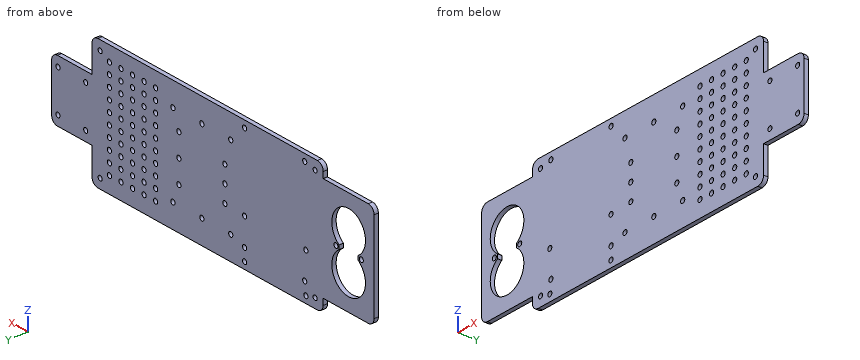
from build123d import *

# Parameters (mm, degrees)
SKETCH1_W           = 200
SKETCH1_H           = 95
BOSS_EXTRUDE1_DEPTH = 3.175
SKETCH3_R           = 1.75
CUT_EXTRUDE2_DEPTH  = 118.785400915
SKETCH4_W           = 76
SKETCH4_H           = 3.175
BOSS_EXTRUDE2_DEPTH = 44
SKETCH5_R           = 1.75
CUT_EXTRUDE3_DEPTH  = 148.223024992
SKETCH7_W           = 45
SKETCH7_H           = 3.175
BOSS_EXTRUDE3_DEPTH = 35
SKETCH8_R           = 1.75
CUT_EXTRUDE4_DEPTH  = 151.064564226
FILLET1_R           = 5
SKETCH9_R           = 1.775
CUT_EXTRUDE5_DEPTH  = 151.064564226
SKETCH10_R          = 1.8
SKETCH10_R_2        = 1.775
CUT_EXTRUDE6_DEPTH  = 151.064564226
SKETCH11_R          = 1.8
CUT_EXTRUDE7_DEPTH  = 151.064564226
SKETCH12_R          = 1.8
CUT_EXTRUDE8_DEPTH  = 151.064564226


with BuildPart() as part:
    # Sketch1 → Boss-Extrude1 (new body)
    with BuildSketch(Plane(origin=(0, 0, 0), x_dir=(1, 0, 0), z_dir=(0, 1, 0))):
        with Locations((6.013896682, 3.728641929)):
            Rectangle(SKETCH1_W, SKETCH1_H)
    extrude(amount=BOSS_EXTRUDE1_DEPTH)

    # Sketch3 → Cut-Extrude2 (cut, through all)
    with BuildSketch(Plane(origin=(0, 3.175, 0), x_dir=(1, 0, 0), z_dir=(0, 1, 0))):
        with Locations(Location((-86.986103318, -36.771358071, 0), (0, 0, 270))):
            Circle(SKETCH3_R)
        with Locations(Location((-86.986103318, 44.228641929, 0), (0, 0, 270))):
            Circle(SKETCH3_R)
        with Locations(Location((99.013896682, 44.228641929, 0), (0, 0, 270))):
            Circle(SKETCH3_R)
        with Locations(Location((99.013896682, -36.771358071, 0), (0, 0, 270))):
            Circle(SKETCH3_R)
    extrude(amount=-CUT_EXTRUDE2_DEPTH, mode=Mode.SUBTRACT)

    # Sketch4 → Boss-Extrude2 (add)
    with BuildSketch(Plane.ZY.offset(93.986103318)):
        with Locations((-3.728641929, 1.5875)):
            Rectangle(SKETCH4_W, SKETCH4_H)
    extrude(amount=BOSS_EXTRUDE2_DEPTH)

    # Sketch5 → Cut-Extrude3 (cut, through all)
    with BuildSketch(Plane(origin=(0, 3.175, 0), x_dir=(1, 0, 0), z_dir=(0, 1, 0))):
        with Locations(Location((-126.986103318, 3.728641929, 0), (0, 0, 270))):
            Circle(SKETCH5_R)
        with Locations(Location((-104.986103318, 3.728641929, 0), (0, 0, 270))):
            Circle(SKETCH5_R)
        with BuildLine():
            Line((-124.286103318, 2.179060332), (-124.286103318, 5.278223526))
            ThreePointArc((-124.286103318, 5.278223526), (-115.986103318, 31.778641929), (-107.686103318, 5.278223526))
            Line((-107.686103318, 5.278223526), (-107.686103318, 2.179060332))
            ThreePointArc((-107.686103318, 2.179060332), (-115.986103318, -24.321358071), (-124.286103318, 2.179060332))
        make_face()
    extrude(amount=-CUT_EXTRUDE3_DEPTH, mode=Mode.SUBTRACT)

    # Sketch7 → Boss-Extrude3 (add)
    with BuildSketch(Plane(origin=(106.013896682, 0, 0), x_dir=(0, 0, -1), z_dir=(1, 0, 0))):
        with Locations((3.728641929, 1.5875)):
            Rectangle(SKETCH7_W, SKETCH7_H)
    extrude(amount=BOSS_EXTRUDE3_DEPTH)

    # Sketch8 → Cut-Extrude4 (cut, through all)
    with BuildSketch(Plane(origin=(0, 3.175, 0), x_dir=(1, 0, 0), z_dir=(0, 1, 0))):
        with Locations(Location((111.513896682, -11.471358071, 0), (0, 0, 270))):
            Circle(SKETCH8_R)
        with Locations(Location((111.513896682, 18.928641929, 0), (0, 0, 270))):
            Circle(SKETCH8_R)
        with Locations(Location((135.513896682, -11.471358071, 0), (0, 0, 270))):
            Circle(SKETCH8_R)
        with Locations(Location((135.513896682, 18.928641929, 0), (0, 0, 270))):
            Circle(SKETCH8_R)
    extrude(amount=-CUT_EXTRUDE4_DEPTH, mode=Mode.SUBTRACT)

    # Fillet1
    fillet1_edges = [part.edges().sort_by_distance(p)[0] for p in [
        (106.013896682, 1.5875, -51.228641929),
        (141.013896682, 1.5875, -26.228641929),
        (141.013896682, 1.5875, 18.771358071),
        (106.013896682, 1.5875, 43.771358071),
        (-93.986103318, 1.5875, -51.228641929),
        (-93.986103318, 1.5875, 43.771358071),
        (-137.986103318, 1.5875, -41.728641929),
        (-137.986103318, 1.5875, 34.271358071),
    ]]
    fillet(fillet1_edges, radius=FILLET1_R)

    # Sketch9 → Cut-Extrude5 (cut, through all)
    with BuildSketch(Plane(origin=(0, 3.175, 0), x_dir=(1, 0, 0), z_dir=(0, 1, 0))):
        with Locations(Location((-78.986103318, 46.228641929, 0), (0, 0, 270))):
            Circle(SKETCH9_R)
        with Locations(Location((-25.986103318, 46.228641929, 0), (0, 0, 270))):
            Circle(SKETCH9_R)
        with Locations(Location((-25.986103318, 17.228641929, 0), (0, 0, 270))):
            Circle(SKETCH9_R)
        with Locations(Location((-78.986103318, 17.228641929, 0), (0, 0, 270))):
            Circle(SKETCH9_R)
    extrude(amount=-CUT_EXTRUDE5_DEPTH, mode=Mode.SUBTRACT)

    # Sketch10 → Cut-Extrude6 (cut, through all)
    with BuildSketch(Plane(origin=(0, 3.175, 0), x_dir=(1, 0, 0), z_dir=(0, 1, 0))):
        with Locations(Location((-13.986103318, 33.728641929, 0), (0, 0, 270))):
            Circle(SKETCH10_R)
        with Locations(Location((11.013896682, 33.728641929, 0), (0, 0, 270))):
            Circle(SKETCH10_R)
        with Locations(Location((36.013896682, 33.728641929, 0), (0, 0, 270))):
            Circle(SKETCH10_R)
        with Locations(Location((-13.986103318, -26.271358071, 0), (0, 0, 270))):
            Circle(SKETCH10_R)
        with Locations(Location((11.013896682, -26.271358071, 0), (0, 0, 270))):
            Circle(SKETCH10_R)
        with Locations(Location((36.013896682, -26.271358071, 0), (0, 0, 270))):
            Circle(SKETCH10_R)
        with Locations(Location((-8.886103318, 3.728641929, 0), (0, 0, 270))):
            Circle(SKETCH10_R)
        with Locations(Location((30.913896682, 3.728641929, 0), (0, 0, 270))):
            Circle(SKETCH10_R)
        with Locations(Location((-8.886103318, 16.228641929, 0), (0, 0, 270))):
            Circle(SKETCH10_R_2)
        with Locations(Location((-8.886103318, -8.771358071, 0), (0, 0, 270))):
            Circle(SKETCH10_R_2)
        with Locations(Location((30.913896682, -13.071358071, 0), (0, 0, 270))):
            Circle(SKETCH10_R)
        with Locations(Location((30.913896682, 20.528641929, 0), (0, 0, 270))):
            Circle(SKETCH10_R)
    extrude(amount=-CUT_EXTRUDE6_DEPTH, mode=Mode.SUBTRACT)

    # Sketch11 → Cut-Extrude7 (cut, through all)
    with BuildSketch(Plane(origin=(0, 3.175, 0), x_dir=(1, 0, 0), z_dir=(0, 1, 0))):
        with Locations(Location((-77.986103318, 37.228641929, 0), (0, 0, 270))):
            Circle(SKETCH11_R)
        with Locations(Location((-25.986103318, 37.228641929, 0), (0, 0, 270))):
            Circle(SKETCH11_R)
        with Locations(Location((-77.986103318, -38.671358071, 0), (0, 0, 270))):
            Circle(SKETCH11_R)
        with Locations(Location((-25.986103318, -38.671358071, 0), (0, 0, 270))):
            Circle(SKETCH11_R)
    extrude(amount=-CUT_EXTRUDE7_DEPTH, mode=Mode.SUBTRACT)

    # Sketch12 → Cut-Extrude8 (cut, through all)
    with BuildSketch(Plane(origin=(0, 3.175, 0), x_dir=(1, 0, 0), z_dir=(0, 1, 0))):
        with Locations(Location((51.013896682, 39.228641929, 0), (0, 0, 270))):
            Circle(SKETCH12_R)
        with Locations(Location((51.013896682, 31.228641929, 0), (0, 0, 270))):
            Circle(SKETCH12_R)
        with Locations(Location((51.013896682, 23.228641929, 0), (0, 0, 270))):
            Circle(SKETCH12_R)
        with Locations(Location((51.013896682, 15.228641929, 0), (0, 0, 270))):
            Circle(SKETCH12_R)
        with Locations(Location((51.013896682, 7.228641929, 0), (0, 0, 270))):
            Circle(SKETCH12_R)
        with Locations(Location((51.013896682, -0.771358071, 0), (0, 0, 270))):
            Circle(SKETCH12_R)
        with Locations(Location((51.013896682, -8.771358071, 0), (0, 0, 270))):
            Circle(SKETCH12_R)
        with Locations(Location((51.013896682, -16.771358071, 0), (0, 0, 270))):
            Circle(SKETCH12_R)
        with Locations(Location((51.013896682, -24.771358071, 0), (0, 0, 270))):
            Circle(SKETCH12_R)
        with Locations(Location((51.013896682, -32.771358071, 0), (0, 0, 270))):
            Circle(SKETCH12_R)
        with Locations(Location((61.013896682, 31.228641929, 0), (0, 0, 270))):
            Circle(SKETCH12_R)
        with Locations(Location((61.013896682, 23.228641929, 0), (0, 0, 270))):
            Circle(SKETCH12_R)
        with Locations(Location((61.013896682, 15.228641929, 0), (0, 0, 270))):
            Circle(SKETCH12_R)
        with Locations(Location((61.013896682, 7.228641929, 0), (0, 0, 270))):
            Circle(SKETCH12_R)
        with Locations(Location((61.013896682, -0.771358071, 0), (0, 0, 270))):
            Circle(SKETCH12_R)
        with Locations(Location((61.013896682, -8.771358071, 0), (0, 0, 270))):
            Circle(SKETCH12_R)
        with Locations(Location((61.013896682, -16.771358071, 0), (0, 0, 270))):
            Circle(SKETCH12_R)
        with Locations(Location((61.013896682, -24.771358071, 0), (0, 0, 270))):
            Circle(SKETCH12_R)
        with Locations(Location((61.013896682, -32.771358071, 0), (0, 0, 270))):
            Circle(SKETCH12_R)
        with Locations(Location((71.013896682, 31.228641929, 0), (0, 0, 270))):
            Circle(SKETCH12_R)
        with Locations(Location((71.013896682, 23.228641929, 0), (0, 0, 270))):
            Circle(SKETCH12_R)
        with Locations(Location((71.013896682, 15.228641929, 0), (0, 0, 270))):
            Circle(SKETCH12_R)
        with Locations(Location((71.013896682, 7.228641929, 0), (0, 0, 270))):
            Circle(SKETCH12_R)
        with Locations(Location((71.013896682, -0.771358071, 0), (0, 0, 270))):
            Circle(SKETCH12_R)
        with Locations(Location((71.013896682, -8.771358071, 0), (0, 0, 270))):
            Circle(SKETCH12_R)
        with Locations(Location((71.013896682, -16.771358071, 0), (0, 0, 270))):
            Circle(SKETCH12_R)
        with Locations(Location((71.013896682, -24.771358071, 0), (0, 0, 270))):
            Circle(SKETCH12_R)
        with Locations(Location((71.013896682, -32.771358071, 0), (0, 0, 270))):
            Circle(SKETCH12_R)
        with Locations(Location((81.013896682, 31.228641929, 0), (0, 0, 270))):
            Circle(SKETCH12_R)
        with Locations(Location((81.013896682, 23.228641929, 0), (0, 0, 270))):
            Circle(SKETCH12_R)
        with Locations(Location((81.013896682, 15.228641929, 0), (0, 0, 270))):
            Circle(SKETCH12_R)
        with Locations(Location((81.013896682, 7.228641929, 0), (0, 0, 270))):
            Circle(SKETCH12_R)
        with Locations(Location((81.013896682, -0.771358071, 0), (0, 0, 270))):
            Circle(SKETCH12_R)
        with Locations(Location((81.013896682, -8.771358071, 0), (0, 0, 270))):
            Circle(SKETCH12_R)
        with Locations(Location((81.013896682, -16.771358071, 0), (0, 0, 270))):
            Circle(SKETCH12_R)
        with Locations(Location((81.013896682, -24.771358071, 0), (0, 0, 270))):
            Circle(SKETCH12_R)
        with Locations(Location((81.013896682, -32.771358071, 0), (0, 0, 270))):
            Circle(SKETCH12_R)
        with Locations(Location((91.013896682, 31.228641929, 0), (0, 0, 270))):
            Circle(SKETCH12_R)
        with Locations(Location((91.013896682, 23.228641929, 0), (0, 0, 270))):
            Circle(SKETCH12_R)
        with Locations(Location((91.013896682, 15.228641929, 0), (0, 0, 270))):
            Circle(SKETCH12_R)
        with Locations(Location((91.013896682, 7.228641929, 0), (0, 0, 270))):
            Circle(SKETCH12_R)
        with Locations(Location((91.013896682, -0.771358071, 0), (0, 0, 270))):
            Circle(SKETCH12_R)
        with Locations(Location((91.013896682, -8.771358071, 0), (0, 0, 270))):
            Circle(SKETCH12_R)
        with Locations(Location((91.013896682, -16.771358071, 0), (0, 0, 270))):
            Circle(SKETCH12_R)
        with Locations(Location((91.013896682, -24.771358071, 0), (0, 0, 270))):
            Circle(SKETCH12_R)
        with Locations(Location((91.013896682, -32.771358071, 0), (0, 0, 270))):
            Circle(SKETCH12_R)
        with Locations(Location((61.013896682, 39.228641929, 0), (0, 0, 270))):
            Circle(SKETCH12_R)
        with Locations(Location((71.013896682, 39.228641929, 0), (0, 0, 270))):
            Circle(SKETCH12_R)
        with Locations(Location((81.013896682, 39.228641929, 0), (0, 0, 270))):
            Circle(SKETCH12_R)
        with Locations(Location((91.013896682, 39.228641929, 0), (0, 0, 270))):
            Circle(SKETCH12_R)
    extrude(amount=-CUT_EXTRUDE8_DEPTH, mode=Mode.SUBTRACT)


solid = part.part
Geometry: final body of the model. Coordinates: model frame, mm. Round coordinates to 2 decimals unless told otherwise and drop trailing zeros. Loops run counter-clockwise (first coordinate to the right, second up) from the corner with the lowest first, then second, coordinate; pieces in that order, holes last. Notation, with made-up numbers: (75, -37) - (87, -37) arc R20 cw to (87, -10) - close; hole circle Ø8 at (83, 35.25). An arc over 180 degrees is marked (long way). Write each question's results on one line, items separated by ' | '. Start each with the question number.
1) Cut plane B-B on y = 1.1. Count the separate pieces of the cut face and the enclosed holes in it, then the cut area to 3 significant figures.
2) Cut plane A-A on x = -119.5. Return loops of the section in (y, z) (3 decimals).
3) First-contact query: P1, Ø3, axis at x = 71.01, z = -15.23, coming from the -Y side; P2, Ø1, axis at y = 1, z = -39, coming from the +X side. Flat tips, straight axial feed; report the tip coordinate or a pass-through.
4) Line query: probe 1 along X at (y, z) = (2.8, 12); probe 2 along X at (y, z) = (2.75, 13); probe 3 along Z at (x, y) = (-15, 2.15). Output: solid intervals per line, ascending. Write a range as [from, to].
Verdict:
1) separate pieces: 1 | enclosed holes: 81 | area: 21,700 mm2
2) outline: (0, -41.729) - (3.175, -41.729) - (3.175, -31.348) - (0, -31.348) - close; (0, 23.891) - (3.175, 23.891) - (3.175, 34.271) - (0, 34.271) - close
3) P1: passes through | P2: stops at x = 106.01
4) probe 1: x = [-137.99, -130.36], [-101.61, 29.47], [32.36, 109.85], [113.18, 133.85], [137.18, 141.01] | probe 2: x = [-137.99, -130.17], [-101.8, 29.12], [32.71, 110.66], [112.37, 134.66], [136.37, 141.01] | probe 3: z = [-51.23, -35.22], [-32.24, 24.78], [27.76, 43.77]
